Could you check a few things on this model? Use its own coordinates, in mm. A direction names the side the tool comes from. Round coordinates to 2 decimals unless told otherwise and drop trailing zeros. Write each loop counter-clockwise with the first axis right and the second up, starting at its lowest first coordinate (ties: lowest second). Pieces come first, ordered by that corner, then holes. Notation, with made-up numbers: (66.5, 13.5) -> (73.5, 13.5) arc R17 cw to (73.5, 46.5) -> close; hole circle Ø2 at (55.5, 9). An arc over 180 degrees is marked (long way). Return JSON: item names as keys, results as strings.
Solid Edge part; units mm, degrees
sketch "Sketch1" plane through (0, 0, 0) normal (0, -1, 0) x (1, 0, 0)
  line L0 (-39.896, 10) -> (30.104, 10)
  line L1 (-39.896, -10) -> (30.104, -10)
  line L2 (-39.896, -10) -> (-39.896, -22.5)
  line L3 (-99.896, -22.5) -> (-39.896, -22.5)
  line L4 (-99.896, -10) -> (-99.896, -22.5)
  line L5 (-99.896, -10) -> (-99.896, -6.077)
  line L6 (-99.896, -6.077) -> (-39.896, 10)
  arc A0 (30.104, 10) -> (30.104, -10) centre (30.104, 0) cw
  circle A1 centre (30.104, 0) radius 5
  circle A2 centre (0, 0) radius 5
  dimension "D1" = 39.896
  dimension "D2" = 39.896
  dimension "D3" = 39.896
  dimension "D4" = 99.896
extrude "Protrusion1" add sketch "Sketch1" along normal mid plane 4
hole "Agujero_1" at (-79.896, 0, -22.5) direction (0, 0, 1) diameter 2.459 depth 6 tip angle 118 thread major 3 thread length 5
hole "Hole1" at (-44.896, 0, -22.5) direction (0, 0, 1) diameter 2.459 depth 6 tip angle 118 thread major 3 thread length 5
properties part number "1976-1500-005" material "Aluminio, 7075-T6"
1) If I drill on probe 1 along X at (y, z) = (0, -20.1); probe 2 along X at (y, z) = (0.5, -20.5); probe 3 along Z at (x, y) = (15, -1.55), over which ranges is the centre line in solid material (lowest first)? Write a range as [from, to].
Return value:
{"probe 1": "[-99.9, -81.13], [-78.67, -46.13], [-43.67, -39.9]", "probe 2": "[-99.9, -81.02], [-78.77, -46.02], [-43.77, -39.9]", "probe 3": "[-10, 10]"}
2) Thinking about a two-plate mould opening in Y: for faces 4 (the face through (-44, 2, -6)), 5 (the face through (-44, -2, -6)), 6 (the face through (-80.933, 0.661, -19.458)), 7 (the face through (-70, 0, -22.5)), which applies, pulls with the +Y half, pulls with the -Y half, needs draft (parallel to the pull), parting line crosses it, or undercut?
Return value:
{"face 4": "pulls with the +Y half", "face 5": "pulls with the -Y half", "face 6": "undercut", "face 7": "needs draft"}
3) I want a section at B-B, the plane z = 0. Please give me the cut outline in (x, y), and give its area (3 significant figures).
Return value:
{"outline": "(-77.22, -2) -> (-5, -2) -> (-5, 2) -> (-77.22, 2) -> close; (5, -2) -> (25.1, -2) -> (25.1, 2) -> (5, 2) -> close; (35.1, -2) -> (40.1, -2) -> (40.1, 2) -> (35.1, 2) -> close", "area": "389 mm²"}
4) I want a section at C-C, the plane z = -20. Please give me the cut outline in (x, y).
Return value:
{"outline": "(-99.9, -2) -> (-39.9, -2) -> (-39.9, 2) -> (-99.9, 2) -> close; hole circle Ø2.46 at (-79.9, 0); hole circle Ø2.46 at (-44.9, 0)"}
5) I want a section at A-A, the plane x = 0. Please give me the cut outline in (y, z).
Return value:
{"outline": "(-2, -10) -> (2, -10) -> (2, -5) -> (-2, -5) -> close; (-2, 5) -> (2, 5) -> (2, 10) -> (-2, 10) -> close"}
6) For faces 1 (the face through (-43.805, 0.567, -19.458)), 2 (the face through (-39.896, 0, -16)), 3 (the face through (-70.316, 0.028, 1.849)), which set-ups out of +Z, -Z, +X, -X, +Y, -Y let a thin tool reach every point of the face, with its end or its side?
Return value:
{"face 1": "-Z", "face 2": "-Z, +X, +Y, -Y", "face 3": "+Z, -X, +Y, -Y"}
7) I want a section at D-D, the plane x = -31. Please give me the cut outline in (y, z).
Return value:
{"outline": "(-2, -10) -> (2, -10) -> (2, 10) -> (-2, 10) -> close"}
8) Will these pins go through, and if not, where does the flat tip stop? pin 1 Ø1.2 at (y, z) = (-0.5, -16.5) entering from +X; pin 2 Ø2 at (x, y) = (7.5, 0) entering from -Z; pin 3 Ø1.5 at (x, y) = (-44.896, 0) entering from +Z; pin 4 Ø9 at (x, z) = (30.104, 0) entering from -Y.
Return value:
{"pin 1": "x = -39.9", "pin 2": "z = -10", "pin 3": "z = 8.86", "pin 4": "through"}
